Source: CAD feature listing. Evaluate the final solid. Frame: model axes, mm. Face numbers are marked on the shaded views. A direction names the side the tool comes from. Give positions to 0.01 mm unless a question says otherwise; leave off trailing zeros. Loops run counter-clockwise (first coordinate to the right, second up) from the corner with the lowest first, then second, coordinate; pieces in that order, holes last. Notation, with made-up numbers: (49, 55) - (59, 55) arc R29 ccw to (59, 91) - close; hole circle Ø1 at (-6, -22.5). An arc over 180 degrees is marked (long way). Put each result on its own line as item: value.
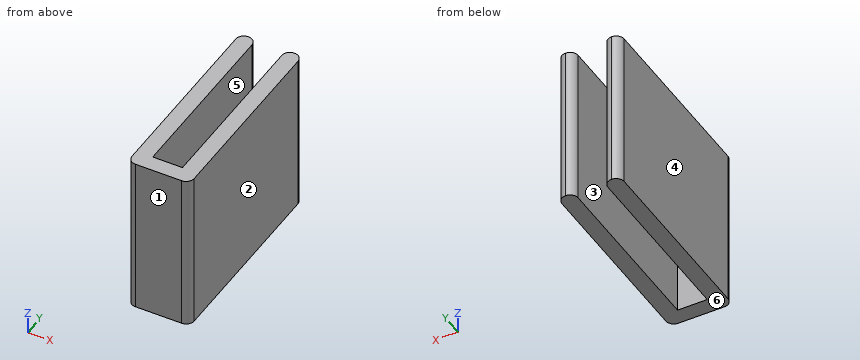
```python
from build123d import *

# Parameters (mm, degrees)
BOSS_EXTRUDE1_DEPTH = 8


with BuildPart() as part:
    # Sketch1 → Boss-Extrude1 (new body)
    with BuildSketch(Plane.XY):
        with BuildLine():
            Line((2.69, 10), (2.7, 10))
            ThreePointArc((2.7, 10), (2.982842712, 9.882842712), (3.1, 9.6))
            Line((3.1, 9.6), (3.1, 0.4))
            ThreePointArc((3.1, 0.4), (2.982842712, 0.117157288), (2.7, 0))
            Line((2.7, 0), (0.4, 0))
            ThreePointArc((0.4, 0), (0.117157288, 0.117157288), (0, 0.4))
            Line((0, 0.4), (0, 9.6))
            ThreePointArc((0, 9.6), (0.117157288, 9.882842712), (0.4, 10))
            Line((0.4, 10), (0.41, 10))
            ThreePointArc((0.41, 10), (0.692842712, 9.882842712), (0.81, 9.6))
            Line((0.81, 9.6), (0.81, 0.8))
            Line((0.81, 0.8), (2.29, 0.8))
            Line((2.29, 0.8), (2.29, 9.6))
            ThreePointArc((2.29, 9.6), (2.407157288, 9.882842712), (2.69, 10))
        make_face()
    extrude(amount=BOSS_EXTRUDE1_DEPTH)


solid = part.part
```
1) Section query A-A, the plane y = 1. Output: boundary loops of the cut face in (x, z), plus the area to 3 significant figures.
Check result:
outline: (0, 0) - (0.81, 0) - (0.81, 8) - (0, 8) - close; (2.29, 0) - (3.1, 0) - (3.1, 8) - (2.29, 8) - close
area: 13.0 mm²
2) Material intervals for line 1 along X through (y, z) = (3.75, 2.5); line 2 along Y through (x, z) = (2.1, 4); line 3 along Y through (x, z) = (0.55, 1.5), sorted ascending. Write a range as [from, to].
Check result:
line 1: [0, 0.81], [2.29, 3.1]
line 2: [0, 0.8]
line 3: [0, 9.97]
3) Access query for the marked faces 5 and 6. Directions: +Z, -Z, +X, -X, +Y, -Y. A direction counts if a zero-diameter tool reaches every point of the face in a straight line with its end or side. Return the directions, or none.
Check result:
face 5: +Z, -Z, +Y
face 6: -Z, +X, -X, +Y, -Y
4) Mould query, pull axis X, two halves, no side actions, for the marked faces 1, 2, 3 and 4. Classes: pulls with the +X half, pulls with the -X half, needs draft (parallel to the pull), parting line crosses it, or undercut.
Check result:
face 1: needs draft
face 2: pulls with the +X half
face 3: undercut
face 4: pulls with the -X half
